Check sheet for the modelled part. Datum: model origin and axes. Units: mm. Round coordinates to 2 decimals unless told otherwise and drop trailing zeros. Write each loop counter-clockwise with the first axis right and the second up, starting at its lowest first coordinate (ties: lowest second). Pieces come first, ordered by that corner, then holes. Notation, with made-up numbers: M 22.5,17.25 L 53.5,17.25 A13 cw 53.5,35.25 Z; hole C 35,47.5 d5. An arc over 180 degrees is marked long. Answer in a Markdown table with one row per item.
Autodesk Inventor part; units mm, degrees
ref_plane "YZ Plane" through (0, 0, 0) normal (1, 0, 0) x (0, 1, 0)
ref_plane "XZ Plane" through (0, 0, 0) normal (0, 1, 0) x (-1, 0, 0)
ref_plane "XY Plane" through (0, 0, 0) normal (0, 0, 1) x (1, 0, 0)
sketch "Sketch1" plane through (0, 0, 0) normal (0, 0, 1) x (1, 0, 0)
  arc A0 (-12.435485, 76.169317) -> (-19.719816, 39.609757) centre (18.622974, 50.975591) ccw
  arc A1 (-12.435485, 76.169317) -> (-8.899951, 72.633783) centre (-2.589145, 82.480123) ccw
  line L0 (-12.435485, 76.169317) -> (-8.899951, 72.633783) construction
  line L1 (-12.435485, 76.169317) -> (-7.435485, 76.169317) construction
  arc A2 (-8.899951, 72.633783) -> (8.917299, 32.302519) centre (65.581671, 81.436509) ccw
  arc A3 (8.917299, 32.302519) -> (3.260445, 26.645665) centre (13.582916, 21.980048) ccw
  line L2 (8.917299, 32.302519) -> (3.260445, 26.645665) construction
  line L3 (8.917299, 32.302519) -> (16.917299, 32.302519) construction
  arc A4 (-19.70552, 35.111295) -> (3.260445, 26.645665) centre (-7.920046, 31.699095) ccw
  arc A5 (-19.70552, 35.111295) -> (-19.719816, 39.609757) centre (-27.389927, 37.336129) ccw
  circle A6 centre (-7.920046, 31.699095) radius 1.5
  line L4 (-21.368921, 76.169317) -> (8.917299, 76.169317)
  line L5 (8.917299, 76.169317) -> (8.917299, 19.429599)
  line L6 (8.917299, 19.429599) -> (-21.368921, 19.429599)
  line L7 (-21.368921, 19.429599) -> (-21.368921, 76.169317)
  line L8 (-21.368921, 39.609757) -> (3.327974, 39.609757)
  line L9 (-19.719816, 39.609757) -> (3.327974, 39.609757) construction
  line L10 (3.327974, 39.609757) -> (3.327974, 76.169317)
  line L11 (3.327974, 39.609757) -> (39.887534, 39.609757) construction
  dimension "d25" = 39.9919
  dimension "d26" = 5
  dimension "d27" = 45
  dimension "d28" = 75
  dimension "d29" = 8
  dimension "d30" = 135
  dimension "d31" = 8
  dimension "d32" = 3
  dimension "d51" = 0
  dimension "d52" = 90
sketch "Sketch1 outline for Extrusion1" plane through (0, 0, 0) normal (0, 0, 1) x (1, 0, 0)
  arc A0 (-8.899951, 72.633783) -> (-12.435485, 76.169317) centre (-2.589145, 82.480123) cw
  arc A1 (8.917299, 32.302519) -> (-8.899951, 72.633783) centre (65.581671, 81.436509) cw
  arc A2 (-12.435485, 76.169317) -> (-19.719816, 39.609757) centre (18.622974, 50.975591) ccw
  arc A3 (3.260445, 26.645665) -> (8.917299, 32.302519) centre (13.582916, 21.980048) cw
  arc A4 (-19.719816, 39.609757) -> (-19.70552, 35.111295) centre (-27.389927, 37.336129) cw
  arc A5 (-19.70552, 35.111295) -> (3.260445, 26.645665) centre (-7.920046, 31.699095) ccw
  circle A6 centre (-7.920046, 31.699095) radius 1.5
extrude "Extrusion1" add sketch "Sketch1 outline for Extrusion1" along normal blind 3
sketch "Sketch2" plane through (0, 0, 0) normal (0, 0, -1) x (-1, 0, 0)
  arc A0 (8.899951, 72.633783) -> (12.435485, 76.169317) centre (2.589145, 82.480123) ccw
  arc A1 (19.719816, 39.609757) -> (12.435485, 76.169317) centre (-18.622974, 50.975591) ccw
  arc A2 (-8.917299, 32.302519) -> (8.899951, 72.633783) centre (-65.581671, 81.436509) ccw
  arc A3 (19.719816, 39.609757) -> (19.70552, 35.111295) centre (27.389927, 37.336129) ccw
  line L0 (19.719816, 39.609757) -> (0.192482, 45.398184)
  arc A4 (11.216243, 74.583931) -> (12.435485, 76.169317) centre (2.589145, 82.480123) ccw
  arc A5 (9.327537, 42.690308) -> (11.216243, 74.583931) centre (-26.326768, 60.804454) ccw
  point P0 (0, 0)
  dimension "d35" = 0
  dimension "d37" = 2
sketch "Sketch2 outline for Extrusion2" plane through (0, 0, 0) normal (0, 0, -1) x (-1, 0, 0)
  arc A0 (19.719816, 39.609757) -> (12.435485, 76.169317) centre (-18.622974, 50.975591) ccw
  line L0 (9.327537, 42.690308) -> (19.719816, 39.609757)
  arc A1 (11.216243, 74.583931) -> (9.327537, 42.690308) centre (-26.326768, 60.804454) cw
  arc A2 (12.435485, 76.169317) -> (11.216243, 74.583931) centre (2.589145, 82.480123) cw
extrude "Extrusion2" add sketch "Sketch2 outline for Extrusion2" against normal blind 3
sketch "Sketch5" plane through (0, 0, 3) normal (0, 0, 1) x (1, 0, 0)
  line L0 (-9.327537, 42.690308) -> (-19.719816, 39.609757)
  line L1 (-9.327537, 42.690308) -> (-9.327537, 72.921318)
  arc A0 (-12.435485, 76.169317) -> (-8.899951, 72.633783) centre (-2.589145, 82.480123) ccw
  line L2 (-9.327537, 42.690308) -> (20.903473, 42.690308) construction
  line L3 (-19.719816, 39.609757) -> (-9.327537, 39.609757)
  line L4 (-19.719816, 39.609757) -> (-9.327537, 39.609757) construction
  line L5 (-9.327537, 39.609757) -> (-9.327537, 42.690308)
  line L6 (-21.368921, 76.169317) -> (-21.368921, 42.690308)
  arc A1 (-12.435485, 76.169317) -> (-19.719816, 39.609757) centre (18.622974, 50.975591) ccw
  line L7 (-19.719816, 39.609757) -> (-21.368921, 39.609757)
  line L8 (-21.368921, 39.609757) -> (-21.368921, 43.268072)
  line L9 (-21.368921, 76.169317) -> (-9.327537, 76.169317)
  line L10 (-9.327537, 72.921318) -> (-9.327537, 76.169317)
  point P0 (0, 0)
  point P1 (-11.216243, 74.583931)
  point P2 (-21.368921, 50.975591)
  dimension "d47" = 90
  dimension "d48" = 0
sketch "Sketch6" plane through (0, 0, 3) normal (0, 0, 1) x (-1, 0, 0)
  line L0 (21.368921, -76.169317) -> (21.368921, -42.690308)
  arc A0 (19.719816, 39.609757) -> (12.435485, 76.169317) centre (-18.622974, 50.975591) ccw
  point P0 (0, 0)
  point P1 (21.368921, 50.975591)
ref_plane "Work Plane3" through (-9.327537, 76.169317, 3) normal (0, 0, -1) x (0, -1, 0)
extrude "Extrusion3" [suppressed]
draft "FaceDraft7" angle 45 pull direction (0, 0, -1) faces at (-13.99815, 74.110283, 1) (-19.580116, 35.602105, 2) (0.992604, 23.266705, 2) (3.667398, 27.457629, 1) fixed edges at (-20.597986, 58.790194, 3) (-19.389968, 37.361551, 3) (-12.163655, 20.186828, 3) (5.572879, 29.990085, 3)
properties part number "Hoja de Corte"
1. Draft check along X on faces 1 (the face through (-7.23, 33.03, 1.48)), 2 (the face through (-9, 43, 0)), 3 (the face through (-2.895, 50.843, 1.479)). Enter one of: +X half, -X half, draft (parallel to the pull), parting line (faces both ways), or undercut.
Found:
| item | result |
|---|---|
| face 1 | undercut |
| face 2 | draft |
| face 3 | +X half |
2. Section check A-A, the plane z = 1.15. Record the cut outline in (x, y), and give its area (3 significant figures).
Found:
| item | result |
|---|---|
| outline | M -17.95,40.14 A9.85 cw -17.93,34.6 A10.42 ccw 1.57,27.41 A13.18 cw 7.68,33.76 A75 cw -8.9,72.63 A11.7 cw -11.28,74.65 A38.14 ccw Z; hole C -7.92,31.7 d3 |
| area | 806 mm2 |
3. Go/stop test with flat-tipped pins: pin 1 (3 mm diameter, centred on x = -8.5, y = 32, fed in from +Z); pin 2 (1 mm diameter, centred on y = 32.5, z = 1, fed in from +X); pin 3 (1.5 mm diameter, centred on x = -12.5, z = 0.5, fed in from +Y). Record where each tip stops, or that it passes through.
Found:
| item | result |
|---|---|
| pin 1 | stops at z = 3 |
| pin 2 | stops at x = 6.51 |
| pin 3 | stops at y = 73.56 |
4. Scan lines: L1, parallel to Y at x = -14, z = 2.6; L2, parallel to X at y = 26.5, z = 0.35; L3, parallel to X at y = 72.5, z = 1. Record each from-to range of solid material in increasing order.
Found:
| item | result |
|---|---|
| L1 | y = 21.51 to 73.41 |
| L2 | x = -16.01 to 0.17 |
| L3 | x = -12.68 to -8.88 |
